```python
from build123d import *

# Parameters (mm, degrees)
SKETCH1_R           = 20
SKETCH1_R_2         = 4.2
BOSS_EXTRUDE1_DEPTH = 35
SKETCH2_W           = 2
SKETCH2_H           = 25
CUT_EXTRUDE1_DEPTH  = 35
SKETCH4_R           = 1.75
CUT_EXTRUDE2_DEPTH  = 40
CUT_EXTRUDE3_DEPTH  = 11
SKETCH6_R           = 3
CUT_EXTRUDE4_DEPTH  = 11
SKETCH7_R           = 4.35
SKETCH7_R_2         = 3.1
BOSS_EXTRUDE2_DEPTH = 35
SKETCH8_W           = 2
SKETCH8_H           = 8.930849086
CUT_EXTRUDE5_DEPTH  = 50


with BuildPart() as part:
    # Sketch1 → Boss-Extrude1 (new, symmetric)
    with BuildSketch(Plane(origin=(0, 0, 0), x_dir=(1, 0, 0), z_dir=(0, 1, 0))):
        with Locations(Location((0, 0, 0), (0, 0, 270))):
            Circle(SKETCH1_R)
        with Locations(Location((0, 0, 0), (0, 0, 270))):
            Circle(SKETCH1_R_2, mode=Mode.SUBTRACT)
    extrude(amount=BOSS_EXTRUDE1_DEPTH, both=True)

    # Sketch2 → Cut-Extrude1 (cut, symmetric)
    with BuildSketch(Plane(origin=(0, 0, 0), x_dir=(1, 0, 0), z_dir=(0, 1, 0))):
        with Locations((0, 12.5)):
            Rectangle(SKETCH2_W, SKETCH2_H)
    extrude(amount=CUT_EXTRUDE1_DEPTH, both=True, mode=Mode.SUBTRACT)

    # Sketch4 → Cut-Extrude2 (cut)
    with BuildSketch(Plane(origin=(20, 0, 0), x_dir=(0, 0, -1), z_dir=(1, 0, 0))):
        with Locations((10.231687805, 28.75)):
            Circle(SKETCH4_R)
        with Locations((10.231687805, 9.583333333)):
            Circle(SKETCH4_R)
        with Locations((10.231687805, -9.583333333)):
            Circle(SKETCH4_R)
        with Locations((10.231687805, -28.75)):
            Circle(SKETCH4_R)
    extrude(amount=-CUT_EXTRUDE2_DEPTH, mode=Mode.SUBTRACT)

    # Sketch5 → Cut-Extrude3 (cut)
    with BuildSketch(Plane(origin=(20, 0, 0), x_dir=(0, 0, -1), z_dir=(1, 0, 0))):
        Polygon((7.306687805, 7.894583798), (10.231687805, 6.20583426), (13.156687805, 7.894583798), (13.156687805, 11.272082872), (10.231687805, 12.96083241), (7.306687805, 11.272082872), align=None)
        Polygon((10.231687805, 32.127499075), (7.306687805, 30.438749537), (7.306687805, 27.061250463), (10.231687805, 25.372500925), (13.156687805, 27.061250463), (13.156687805, 30.438749537), align=None)
        Polygon((7.306687805, -11.272082868), (10.231687805, -12.960832405), (13.156687805, -11.272082868), (13.156687805, -7.894583793), (10.231687805, -6.205834255), (7.306687805, -7.894583793), align=None)
        Polygon((7.306687805, -30.438749533), (10.231687805, -32.12749907), (13.156687805, -30.438749533), (13.156687805, -27.061250458), (10.231687805, -25.37250092), (7.306687805, -27.061250458), align=None)
    extrude(amount=-CUT_EXTRUDE3_DEPTH, mode=Mode.SUBTRACT)

    # Sketch6 → Cut-Extrude4 (cut)
    with BuildSketch(Plane(origin=(-20, 0, 0), x_dir=(0, 0, -1), z_dir=(1, 0, 0))):
        with Locations(Location((10.231687805, 28.75, 0), (0, 0, 180))):
            Circle(SKETCH6_R)
        with Locations(Location((10.231687805, 9.583333333, 0), (0, 0, 180))):
            Circle(SKETCH6_R)
        with Locations(Location((10.231687805, -9.583333333, 0), (0, 0, 180))):
            Circle(SKETCH6_R)
        with Locations(Location((10.231687805, -28.75, 0), (0, 0, 180))):
            Circle(SKETCH6_R)
    extrude(amount=CUT_EXTRUDE4_DEPTH, mode=Mode.SUBTRACT)

    # Sketch7 → Boss-Extrude2 (add)
    with BuildSketch(Plane.XZ.offset(35)):
        Circle(SKETCH7_R)
        with Locations(Location((0, 0, 0), (0, 0, 270))):
            Circle(SKETCH7_R_2, mode=Mode.SUBTRACT)
    extrude(amount=-BOSS_EXTRUDE2_DEPTH)

    # Sketch8 → Cut-Extrude5 (cut)
    with BuildSketch(Plane.XZ.offset(35)):
        with Locations((0, -5.775706359)):
            Rectangle(SKETCH8_W, SKETCH8_H)
    extrude(amount=-CUT_EXTRUDE5_DEPTH, mode=Mode.SUBTRACT)


solid = part.part
```
Here's how the part is built. I have some questions about the finished solid (model axes, mm). A direction names the side the tool comes from. Give positions to 0.01 mm unless a question says otherwise; leave off trailing zeros. Write each loop counter-clockwise with the first axis right and the second up, starting at its lowest first coordinate (ties: lowest second). Pieces come first, ordered by that corner, then holes. Notation, with made-up numbers: M 14,31 L 41,31 A35 cw 41,68 Z; hole C 80.5,-27.75 d4. An arc over 180 degrees is marked long. Put each result on its own line as item: value. Start each with the question number.
Item 1: If we section it at C-C, the plane y = -28.75: Write out the boundary of the cut face in (x, z).
Item 2: I need wall thicknesses on L1, parallel to X at y = 18.5, z = 0; L2, parallel to X at y = 9, z = -8; L3, parallel to Y at x = -17, z = -9. Which ranges of each line are inside material? Lowest first, please. Write a range as from..to.
Item 3: If we section it at D-D, the plane y = 19: Write out the boundary of the cut face in (x, z).
Item 4: Thinking about a two-plate mould opening in Y: for faces 1 (the cylindrical face through (-0.171, 17.255, 4.197)), 2 (the flat face through (13.88, 12.13, -8.79)), 3 (the flat face through (-4, 35, 4)), which applies, +Y half, -Y half, draft (parallel to the pull), parting line (faces both ways), or undercut?
Item 5: Will these pins go through, and if not, where does the flat tip stop? pin 1 (1 mm diameter, centred on x = 11, y = 28.5, fed in from +Z); pin 2 (8 mm diameter, centred on x = 4.5, y = 25, fed in from +Z); pin 3 (1 mm diameter, centred on x = 16, y = -9.5, fed in from -Z).
Item 6: If we section it at B-B, the plane x = 8: Write out the boundary of the cut face in (y, z).
Item 7: On a 3-axis mill with a long thin cutter (end or side, diameter ignored), from which of +Z, -Z, +X, -X, +Y, -Y can I reach the whole of each face in a straight line? I mean faces 4 (the cylindrical face through (0.1, -17.7, 3.1)), 5 (the flat face through (14, -29, -7.307)), 6 (the flat face through (-9, -8, -9)). Say none if no direction works.
Item 8: If we section it at A-A, the plane z = 0: Write out the boundary of the cut face in (x, y).
Values:
1. outline: M -18.65,-7.23 L -9,-7.23 L -9,-8.48 L -1,-8.48 L -1,-2.93 A3.1 cw long 1,-2.93 L 1,-8.48 L 9,-8.48 L 9,-7.31 L 18.62,-7.31 A20 ccw long Z; M -15,-13.23 A20 ccw -1,-19.97 L -1,-11.98 L -9,-11.98 L -9,-13.23 Z; M 1,-19.97 A20 ccw 15.06,-13.16 L 9,-13.16 L 9,-11.98 L 1,-11.98 Z
2. L1: -20..-4.2, 4.2..20
2. L2: -9..-1, 1..9
2. L3: -35..-31.49, -26.01..-12.32, -6.85..6.85, 12.32..26.01, 31.49..35
3. outline: M -1,-19.97 L -1,-4.08 A4.2 cw long 1,-4.08 L 1,-19.97 A20 ccw long Z
4. face 1: draft
4. face 2: undercut
4. face 3: +Y half
5. pin 1: z = 17.02
5. pin 2: z = 19.99
5. pin 3: z = -7.31
6. outline: M -35,-18.33 L 35,-18.33 L 35,18.33 L -35,18.33 Z; hole C -28.75,-10.23 d3.5; hole C -9.58,-10.23 d3.5; hole C 9.58,-10.23 d3.5; hole C 28.75,-10.23 d3.5
7. face 4: +Y, -Y
7. face 5: +X
7. face 6: -X
8. outline: M -20,-35 L -3.1,-35 L -3.1,0 L -4.2,0 L -4.2,35 L -20,35 Z; M 3.1,-35 L 20,-35 L 20,35 L 4.2,35 L 4.2,0 L 3.1,0 Z
